Verification items for the finished model (mm, model axes). A direction names the side the tool comes from. Coordinates: 2 decimals unless noted, no trailing zeros. Write each loop counter-clockwise with the first axis right and the second up, starting at its lowest first coordinate (ties: lowest second). Pieces come first, ordered by that corner, then holes. Notation, with made-up numbers: M 48,68.25 L 55,68.25 A27 cw 55,104.25 Z; hole C 42,14.5 d4. An arc over 180 degrees is marked long. One line per item, written item: value.
```python
from build123d import *

# Parameters (mm, degrees)
BOSS_EXTRUDE1_DEPTH = 10
CUT_EXTRUDE1_DEPTH  = 9
SKETCH5_R           = 1.5
CUT_EXTRUDE2_DEPTH  = 2
BOSS_EXTRUDE2_DEPTH = 3
SKETCH7_R           = 24.910226266
CUT_EXTRUDE5_DEPTH  = 4


with BuildPart() as part:
    # Sketch1 → Boss-Extrude1 (new body)
    with BuildSketch(Plane.XY):
        with BuildLine():
            Line((3, 0), (32, 0))
            ThreePointArc((32, 0), (34.121320344, -0.878679656), (35, -3))
            Line((35, -3), (35, -32))
            ThreePointArc((35, -32), (34.121320344, -34.121320344), (32, -35))
            Line((32, -35), (3, -35))
            ThreePointArc((3, -35), (0.878679656, -34.121320344), (0, -32))
            Line((0, -32), (0, -3))
            ThreePointArc((0, -3), (0.878679656, -0.878679656), (3, 0))
        make_face()
    extrude(amount=BOSS_EXTRUDE1_DEPTH)

    # Sketch2 → Cut-Extrude1 (cut)
    with BuildSketch(Plane.XY.offset(10)):
        with BuildLine():
            Line((1.5, -4.5), (1.5, -30.5))
            ThreePointArc((1.5, -30.5), (2.378679656, -32.621320344), (4.5, -33.5))
            Line((4.5, -33.5), (30.5, -33.5))
            ThreePointArc((30.5, -33.5), (32.621320344, -32.621320344), (33.5, -30.5))
            Line((33.5, -30.5), (33.5, -4.5))
            ThreePointArc((33.5, -4.5), (32.621320344, -2.378679656), (30.5, -1.5))
            Line((30.5, -1.5), (4.5, -1.5))
            ThreePointArc((4.5, -1.5), (2.378679656, -2.378679656), (1.5, -4.5))
        make_face()
    extrude(amount=-CUT_EXTRUDE1_DEPTH, mode=Mode.SUBTRACT)

    # Sketch5 → Cut-Extrude2 (cut, through all)
    with BuildSketch(Plane.XY.offset(1)):
        with Locations((7.34, -7.34)):
            Circle(SKETCH5_R)
        with Locations((7.34, -27.66)):
            Circle(SKETCH5_R)
        with Locations((27.66, -27.66)):
            Circle(SKETCH5_R)
        with Locations((27.66, -7.34)):
            Circle(SKETCH5_R)
    extrude(amount=-CUT_EXTRUDE2_DEPTH, mode=Mode.SUBTRACT)

    # Sketch3 → Boss-Extrude2 (add)
    with BuildSketch(Plane.XY.offset(1)):
        Polygon((3.1, -3.1), (3.1, -9.1), (4.1, -9.1), (4.1, -4.1), (9.1, -4.1), (9.1, -3.1), align=None)
        Polygon((30.9, -9.1), (31.9, -9.1), (31.9, -3.1), (25.9, -3.1), (25.9, -4.1), (30.9, -4.1), align=None)
        Polygon((25.9, -30.9), (25.9, -31.9), (31.9, -31.9), (31.9, -25.9), (30.9, -25.9), (30.9, -30.9), align=None)
        Polygon((3.1, -25.9), (3.1, -31.9), (9.1, -31.9), (9.1, -30.9), (4.1, -30.9), (4.1, -25.9), align=None)
    extrude(amount=BOSS_EXTRUDE2_DEPTH)

    # Sketch7 → Cut-Extrude5 (cut)
    with BuildSketch(Plane.XY.offset(10)):
        with Locations((16.498966125, -17.5)):
            Circle(SKETCH7_R)
    extrude(amount=-CUT_EXTRUDE5_DEPTH, mode=Mode.SUBTRACT)


solid = part.part
```
Item 1: Cross-section at A-A, the plane x = 7.34. Enter the section's corners in (y, z).
The answers:
outline: M -35,0 L -29.16,0 L -29.16,1 L -30.9,1 L -30.9,4 L -31.9,4 L -31.9,1 L -33.5,1 L -33.5,6 L -35,6 Z; M -26.16,0 L -8.84,0 L -8.84,1 L -26.16,1 Z; M -5.84,0 L 0,0 L 0,6 L -1.5,6 L -1.5,1 L -3.1,1 L -3.1,4 L -4.1,4 L -4.1,1 L -5.84,1 Z
Item 2: Scan lines: line 1 (X direction, y = -29, z = 3.9); line 2 (Y direction, x = 27.66, z = 0.55); line 3 (X direction, y = -18, z = 2.7). Record each from-to range of solid material in increasing order.
The answers:
line 1: x = 0 to 1.5, 3.1 to 4.1, 30.9 to 31.9, 33.5 to 35
line 2: y = -35 to -29.16, -26.16 to -8.84, -5.84 to 0
line 3: x = 0 to 1.5, 33.5 to 35
Item 3: Draft check along Y on faces 3 (the face through (6, -3.1, 2)), 4 (the face through (0.86, -0.9, 2.96)), 5 (the face through (0.9, -34.14, 2.96)). Enter one of: released by +Y, released by -Y, zero draft, split by the parting line, or undercut.
The answers:
face 3: undercut
face 4: released by +Y
face 5: released by -Y
Item 4: Cross-section at B-B, the plane z = 5.5. Enter the section's corners in (x, y), and give its area (3 significant figures).
The answers:
outline: M 0,-32 A3 ccw 3,-35 L 32,-35 A3 ccw 35,-32 L 35,-3 A3 ccw 32,0 L 3,0 A3 ccw 0,-3 Z; hole M 1.5,-30.5 A3 ccw 4.5,-33.5 L 30.5,-33.5 A3 ccw 33.5,-30.5 L 33.5,-4.5 A3 ccw 30.5,-1.5 L 4.5,-1.5 A3 ccw 1.5,-4.5 Z
area: 201 mm²
Item 5: Access from +Z, -Z, +X, -X, +Y, -Y to the whole of each face (thin tool, end or side, straight path). Record for faces 1 (the face through (8.77, -6.89, 0.51)), 2 (the face through (29, -3.1, 2)).
The answers:
face 1: +Z, -Z
face 2: +Z
Item 6: Go/stop test with flat-tipped pins: P1, Ø1.5, axis at x = 11, y = -19.5, coming from the +Z side; P2, Ø3, axis at x = 7.5, y = -5.5, coming from the +Z side; P3, Ø2.5, axis at x = 7.34, y = -7.34, coming from the -Z side. Record where each tip stops, or that it passes through.
The answers:
P1: stops at z = 1
P2: stops at z = 4
P3: passes through
Item 7: Cross-section at D-D, the plane y = -17. Enter the section's corners in (x, z), and give its area (3 significant figures).
The answers:
outline: M 0,0 L 35,0 L 35,6 L 33.5,6 L 33.5,1 L 1.5,1 L 1.5,6 L 0,6 Z
area: 50.0 mm²
Item 8: Cross-section at C-C, the plane y = -27.66. Enter the section's corners in (x, z).
The answers:
outline: M 0,0 L 5.84,0 L 5.84,1 L 4.1,1 L 4.1,4 L 3.1,4 L 3.1,1 L 1.5,1 L 1.5,6 L 0,6 Z; M 8.84,0 L 26.16,0 L 26.16,1 L 8.84,1 Z; M 29.16,0 L 35,0 L 35,6 L 33.5,6 L 33.5,1 L 31.9,1 L 31.9,4 L 30.9,4 L 30.9,1 L 29.16,1 Z
